Input: part model. Units: mm. Frame: model coordinates. Face numbers are marked on the shaded views. A direction names the side the tool comes from. Round coordinates to 2 decimals unless told otherwise and drop trailing zeros. Loops run counter-clockwise (first coordinate to the right, second up) from the corner with the lowest first, then second, coordinate; pieces in that order, holes last.
(1) Cut plane C-C, the plane z = 9.5. Output: boundary loops of the cut face in (x, y), and give its area (3 significant figures).
(2) First-contact query: pin 1 Ø3 at (x, y) = (1.5, 1) entering from +Z; pin 2 Ø1.5 at (x, y) = (0, 0) entering from -Z. Flat tips, straight axial feed; report the tip coordinate or a pass-through.
(3) Cut plane D-D, the plane x = -2.25. Output: boundary loops of the cut face in (y, z), and give its area (3 significant figures).
(4) Line query: line 1 (Y direction, x = 0, z = 5.5); line 2 (Z direction, x = -1.25, y = -0.65); line 3 (Z direction, x = -1, y = -2.3). Output: solid intervals per line, ascending.
(5) Cut plane A-A, the plane x = 0. Output: boundary loops of the cut face in (y, z).
(6) Access query for the marked faces 1 and 2. Directions: +Z, -Z, +X, -X, +Y, -Y. A direction counts if a zero-diameter tool reaches every point of the face in a straight line with its end or side. Return the directions, or none.
(7) Cut plane B-B, the plane y = 0.65. Output: boundary loops of the cut face in (x, z).
from build123d import *

# Parameters (mm, degrees)
F1_DEPTH = 30
F2_R     = 1.1
F3_DEPTH = 1
F4_R     = 1.5
F5_DEPTH = 5
F6_R     = 1.5
F7_DEPTH = 7


with BuildPart() as f1:
    # F0 (on Top) → F1 (new body)
    with BuildSketch(Plane.XY):
        Polygon((1.5877132403, 2.75), (-1.5877132403, 2.75), (-3.1754264805, 0), (-1.5877132403, -2.75), (1.5877132403, -2.75), (3.1754264805, 0), align=None)
    extrude(amount=F1_DEPTH)

    # F2 (on face) → F3 (join)
    with BuildSketch(Plane.XY.offset(30)):
        Circle(F2_R)
    extrude(amount=F3_DEPTH)

    # F4 (on face) → F5 (join)
    with BuildSketch(Plane.XY.offset(31)):
        Circle(F4_R)
    extrude(amount=F5_DEPTH)

    # F6 (on Top) → F7 (cut)
    with BuildSketch(Plane.XY):
        Circle(F6_R)
    extrude(amount=F7_DEPTH, mode=Mode.SUBTRACT)


solid = f1.part
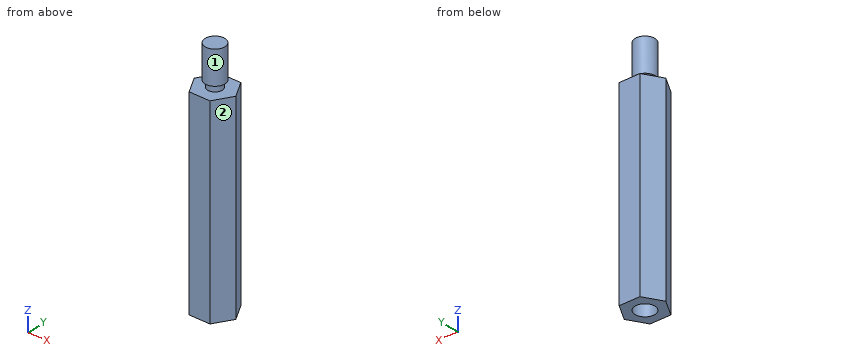
Reported:
1. outline: (-3.18, 0) - (-1.59, -2.75) - (1.59, -2.75) - (3.18, 0) - (1.59, 2.75) - (-1.59, 2.75) - close
1. area: 26.2 mm2
2. pin 1: stops at z = 36
2. pin 2: stops at z = 7
3. outline: (-1.6, 0) - (1.6, 0) - (1.6, 30) - (-1.6, 30) - close
3. area: 96.2 mm2
4. line 1: y = -2.75 to -1.5, 1.5 to 2.75
4. line 2: z = 7 to 30, 31 to 36
4. line 3: z = 0 to 30
5. outline: (-2.75, 0) - (-1.5, 0) - (-1.5, 7) - (1.5, 7) - (1.5, 0) - (2.75, 0) - (2.75, 30) - (1.1, 30) - (1.1, 31) - (1.5, 31) - (1.5, 36) - (-1.5, 36) - (-1.5, 31) - (-1.1, 31) - (-1.1, 30) - (-2.75, 30) - close
6. face 1: +Z
6. face 2: +Z, -Z, +X, -Y
7. outline: (-2.8, 0) - (-1.35, 0) - (-1.35, 7) - (1.35, 7) - (1.35, 0) - (2.8, 0) - (2.8, 30) - (0.89, 30) - (0.89, 31) - (1.35, 31) - (1.35, 36) - (-1.35, 36) - (-1.35, 31) - (-0.89, 31) - (-0.89, 30) - (-2.8, 30) - close
